Work out the finished part from the listing and answer in its coordinate system (mm). Face numbers are marked on the shaded views. A direction names the side the tool comes from. Coordinates: 2 decimals unless noted, no trailing zeros. Order: outer loops, then holes, each group sorted by start corner. A loop starts at its lowest first (then second) coordinate and runs counter-clockwise, first axis right, second up. Notation, with made-up numbers: (-32, 84) -> (-20, 84) arc R10 cw to (-20, 94) -> close; hole circle Ø6 at (-35, -3). An arc over 180 degrees is marked (long way). Use one line per item in the form item = value.
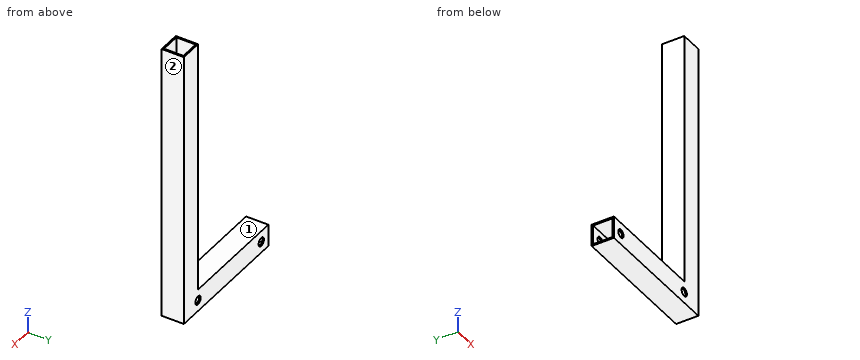
from build123d import *

# Parameters (mm, degrees)
SKETCH1_R           = 4.7625
BOSS_EXTRUDE1_DEPTH = 12.7
SHELL1_T            = -1.651


with BuildPart() as part:
    # Sketch1 → Boss-Extrude1 (new, symmetric)
    with BuildSketch(Plane(origin=(0, 0, 0), x_dir=(1, 0, 0), z_dir=(0, 1, 0))):
        Polygon((-12.7, 12.7), (139.7, 12.7), (139.7, -304.8), (114.3, -304.8), (114.3, -12.7), (-12.7, -12.7), align=None)
        with Locations(Location((0, 0, 0), (0, 0, 270))):
            Circle(SKETCH1_R, mode=Mode.SUBTRACT)
        with Locations(Location((114.3, 0, 0), (0, 0, 270))):
            Circle(SKETCH1_R, mode=Mode.SUBTRACT)
    extrude(amount=BOSS_EXTRUDE1_DEPTH, both=True)

    # Shell1
    shell1_openings = [part.faces().sort_by_distance(p)[0] for p in [
        (127, 0, 304.8),
        (-12.7, 0, 0),
        (0, 0, -4.7625),
        (114.3, 0, -4.7625),
    ]]
    offset(amount=SHELL1_T, openings=shell1_openings, kind=Kind.INTERSECTION)


solid = part.part
(1) Section B-B on z = 0 is taken. Write down the section's boundary in (x, y).
Data:
outline = (-12.7, -12.7) -> (-4.76, -12.7) -> (-4.76, -11.05) -> (-12.7, -11.05) -> close; (-12.7, 11.05) -> (-4.76, 11.05) -> (-4.76, 12.7) -> (-12.7, 12.7) -> close; (4.76, -12.7) -> (109.54, -12.7) -> (109.54, -11.05) -> (4.76, -11.05) -> close; (4.76, 11.05) -> (109.54, 11.05) -> (109.54, 12.7) -> (4.76, 12.7) -> close; (119.06, -12.7) -> (139.7, -12.7) -> (139.7, 12.7) -> (119.06, 12.7) -> (119.06, 11.05) -> (138.05, 11.05) -> (138.05, -11.05) -> (119.06, -11.05) -> close
(2) Each of these flat-tipped pins is pushed along its axis until it touches: P1, Ø6.5, axis at x = 57.5, y = 1.5, coming from the +Z side; P2, Ø7.5, axis at y = 3, z = 156.5, coming from the -X side. Where does it stop, or does it pass through?
Data:
P1 = 12.7
P2 = 114.3
(3) Section A-A on x = 0 is taken. Write down the section's boundary in (y, z), plus the area to 3 significant figures.
Data:
outline = (-12.7, -12.7) -> (12.7, -12.7) -> (12.7, -4.76) -> (11.05, -4.76) -> (11.05, -11.05) -> (-11.05, -11.05) -> (-11.05, -4.76) -> (-12.7, -4.76) -> close; (-12.7, 4.76) -> (-11.05, 4.76) -> (-11.05, 11.05) -> (11.05, 11.05) -> (11.05, 4.76) -> (12.7, 4.76) -> (12.7, 12.7) -> (-12.7, 12.7) -> close
area = 125 mm²
(4) Section C-C on z = 246 is taken. Write down the section's boundary in (x, y).
Data:
outline = (114.3, -12.7) -> (139.7, -12.7) -> (139.7, 12.7) -> (114.3, 12.7) -> close; hole (115.95, -11.05) -> (138.05, -11.05) -> (138.05, 11.05) -> (115.95, 11.05) -> close
(5) Section D-D on y = 5.5 is taken. Write down the section's boundary in (x, z).
Data:
outline = (-12.7, -12.7) -> (139.7, -12.7) -> (139.7, 304.8) -> (138.05, 304.8) -> (138.05, -11.05) -> (-12.7, -11.05) -> close; (-12.7, 11.05) -> (115.95, 11.05) -> (115.95, 304.8) -> (114.3, 304.8) -> (114.3, 12.7) -> (-12.7, 12.7) -> close
(6) Straight lines are drawn through the part: line 1 along X through (y, z) = (12.1, 0); line 2 along Y through (x, z) = (116, 36); line 3 along X through (y, z) = (2.5, 36). For each, find the intervals that lie inside material, in ascending order.
Data:
line_1 = -12.7 to -4.76, 4.76 to 109.54, 119.06 to 139.7
line_2 = -12.7 to -11.05, 11.05 to 12.7
line_3 = 114.3 to 115.95, 138.05 to 139.7
(7) Which of the six approach directions +Z, -Z, +X, -X, +Y, -Y give full straight-line access (tool end or side, diameter ignored) to the marked faces 1 and 2?
Data:
face_1 = +Z, -X, +Y, -Y
face_2 = +Z, -Z, +X, +Y, -Y
